Here's how the part is built. I have some questions about the finished solid (model axes, mm). A direction names the side the tool comes from. Give positions to 0.01 mm unless a question says otherwise; leave off trailing zeros. Order: outer loops, then holes, each group sorted by start corner. A loop starts at its lowest first (then second) coordinate and runs counter-clockwise, first axis right, second up.
from build123d import *

# Parameters (mm, degrees)
ESQUISSE1_W             = 22.3
ESQUISSE1_H             = 43
ESQUISSE1_R             = 2.45
BOSS_EXTRU_1_DEPTH      = 5
BOSS_EXTRU_2_START      = -2.47
ESQUISSE2_R             = 2.45
ESQUISSE2_R_2           = 0.7
BOSS_EXTRU_2_DEPTH      = 2.47
ESQUISSE3_W             = 4
ESQUISSE3_H             = 5
ESQUISSE3_W_2           = 3.94
BOSS_EXTRU_3_DEPTH      = 12.3
ESQUISSE4_R             = 0.7
ENL_V_MAT_EXTRU_1_DEPTH = 52.435201954
BOSS_EXTRU_4_DEPTH      = 2
BOSS_EXTRU_5_DEPTH      = 2
ESQUISSE7_R             = 0.7
BOSS_EXTRU_6_DEPTH      = 4
ESQUISSE8_R             = 0.7
ENL_V_MAT_EXTRU_3_DEPTH = 54.118546667


with BuildPart() as part:
    # Esquisse1 → Boss.-Extru.1 (new body)
    with BuildSketch(Plane.XY):
        with Locations((-11.15, -21.5)):
            Rectangle(ESQUISSE1_W, ESQUISSE1_H)
        with Locations((-6.15, -6.15)):
            Circle(ESQUISSE1_R, mode=Mode.SUBTRACT)
    extrude(amount=BOSS_EXTRU_1_DEPTH)

    # Esquisse2 → Boss.-Extru.2 (add)
    with BuildSketch(Plane.XY.offset(5).offset(BOSS_EXTRU_2_START)):
        with Locations((-6.15, -6.15)):
            Circle(ESQUISSE2_R)
        with Locations((-6.15, -6.15)):
            Circle(ESQUISSE2_R_2, mode=Mode.SUBTRACT)
    extrude(amount=BOSS_EXTRU_2_DEPTH)

    # Esquisse3 → Boss.-Extru.3 (add)
    with BuildSketch(Plane.XY.offset(5)):
        with Locations((-20.3, -40.5)):
            Rectangle(ESQUISSE3_W, ESQUISSE3_H)
        with Locations((-13.54, -40.5)):
            Rectangle(ESQUISSE3_W, ESQUISSE3_H)
        with Locations((-20.3, -12.82)):
            Rectangle(ESQUISSE3_W, ESQUISSE3_H)
        with Locations((-13.57, -12.82)):
            Rectangle(ESQUISSE3_W_2, ESQUISSE3_H)
    extrude(amount=BOSS_EXTRU_3_DEPTH)

    # Esquisse4 → Enlèv. mat.-Extru.1 (cut, through all)
    with BuildSketch(Plane.ZY.offset(22.3)):
        with Locations((11.15, -12.82)):
            Circle(ESQUISSE4_R)
        with Locations((11.15, -40.42)):
            Circle(ESQUISSE4_R)
    extrude(amount=-ENL_V_MAT_EXTRU_1_DEPTH, mode=Mode.SUBTRACT)

    # Esquisse5 → Boss.-Extru.4 (add)
    with BuildSketch(Plane.XZ.offset(43)):
        Polygon((-22.3, 17.3), (-11.54, 17.3), (0, 5), (0, 0), (-22.3, 0), align=None)
    extrude(amount=BOSS_EXTRU_4_DEPTH)

    # Esquisse6 → Boss.-Extru.5 (add)
    with BuildSketch(Plane(origin=(0, -10.32, 0), x_dir=(1, 0, 0), z_dir=(0, 1, 0))):
        Polygon((-22.3, -5), (-22.3, -17.3), (-11.6, -17.3), (0, -5), align=None)
    extrude(amount=BOSS_EXTRU_5_DEPTH)

    # Esquisse7 → Boss.-Extru.6 (add)
    with BuildSketch(Plane(origin=(0, 0, 0), x_dir=(0, 0, -1), z_dir=(1, 0, 0))):
        with BuildLine():
            Line((-11.15, -15.32), (0, -15.32))
            Line((0, -15.32), (0, -27.62))
            Line((0, -27.62), (-11.15, -27.62))
            ThreePointArc((-11.15, -27.62), (-17.3, -21.47), (-11.15, -15.32))
        make_face()
        with Locations(Location((-11.15, -21.47, 0), (0, 0, 90))):
            Circle(ESQUISSE7_R, mode=Mode.SUBTRACT)
    extrude(amount=BOSS_EXTRU_6_DEPTH)

    # Esquisse8 → Enlèv. mat.-Extru.3 (cut, through all)
    with BuildSketch(Plane(origin=(0, 0, 0), x_dir=(-1, 0, 0), z_dir=(0, 0, -1))):
        with Locations((17.3, -40)):
            Circle(ESQUISSE8_R)
        with Locations((5, -40)):
            Circle(ESQUISSE8_R)
        with Locations((5, -20)):
            Circle(ESQUISSE8_R)
        with Locations((17.3, -20)):
            Circle(ESQUISSE8_R)
    extrude(amount=-ENL_V_MAT_EXTRU_3_DEPTH, mode=Mode.SUBTRACT)


solid = part.part
Q1. If we section it at D-D on y = -12.82: List the corners of the cut face in (x, z) for me.
Filled sheet:
outline: (-22.3, 0) - (0, 0) - (0, 5) - (-11.6, 5) - (-11.6, 10.45) - (-15.54, 10.45) - (-15.54, 5) - (-18.3, 5) - (-18.3, 10.45) - (-22.3, 10.45) - close; (-22.3, 11.85) - (-18.3, 11.85) - (-18.3, 17.3) - (-22.3, 17.3) - close; (-15.54, 11.85) - (-11.6, 11.85) - (-11.6, 17.3) - (-15.54, 17.3) - close
Q2. If we section it at A-A on z = 1.5: List the corners of the cut face in (x, y) for me.
Filled sheet:
outline: (-22.3, -45) - (0, -45) - (0, -27.62) - (4, -27.62) - (4, -15.32) - (0, -15.32) - (0, 0) - (-22.3, 0) - close; hole circle Ø1.4 at (-17.3, -40); hole circle Ø1.4 at (-17.3, -20); hole circle Ø4.9 at (-6.15, -6.15); hole circle Ø1.4 at (-5, -40); hole circle Ø1.4 at (-5, -20)
Q3. If we section it at B-B on y = -21.47: List the corners of the cut face in (x, z) for me.
Filled sheet:
outline: (-22.3, 0) - (4, 0) - (4, 10.45) - (0, 10.45) - (0, 5) - (-22.3, 5) - close; (0, 11.85) - (4, 11.85) - (4, 17.3) - (0, 17.3) - close
Q4. Thinking about a two-plate mould opening in Y: for faces 5 (the face through (-11, 0, 2)), 6 (the face through (-9, -22, 0)), 7 (the face through (-4.909, -19.306, 2.465)), which applies, released by +Y, released by -Y, zero draft, split by the parting line, or undercut?
Filled sheet:
face 5: released by +Y
face 6: zero draft
face 7: undercut
Q5. For faces 1 (the face through (-11.6, -11.7, 11.1)), 2 (the face through (-11, -4, 5)), 3 (the face through (-17, -43, 11)), 4 (the face through (-20, -15.32, 11)), which set-ups out of +Z, -Z, +X, -X, +Y, -Y let a thin tool reach every point of the face, with its end or its side?
Filled sheet:
face 1: +Z, +X
face 2: +Z, +X, -X, +Y
face 3: +Z
face 4: +Z, -X
Q6. If we section it at C-C on x = -17.3: List the corners of the cut face in (y, z) for me.
Filled sheet:
outline: (-45, 0) - (-40.7, 0) - (-40.7, 5) - (-43, 5) - (-43, 17.3) - (-45, 17.3) - close; (-39.3, 0) - (-20.7, 0) - (-20.7, 5) - (-39.3, 5) - close; (-19.3, 0) - (0, 0) - (0, 5) - (-8.32, 5) - (-8.32, 17.3) - (-10.32, 17.3) - (-10.32, 5) - (-19.3, 5) - close
Q7. I need wall thicknesses on L1, parallel to Y at x = -17.3, z = 3.25; L2, parallel to Y at x = -21.25, z = 11.15; L3, parallel to X at y = -40, z = 2. Which ranges of each line are inside material? Lowest first, please.
Filled sheet:
L1: y = -45 to -40.7, -39.3 to -20.7, -19.3 to 0
L2: y = -45 to -41.12, -39.72 to -38, -15.32 to -13.52, -12.12 to -8.32
L3: x = -22.3 to -18, -16.6 to -5.7, -4.3 to 0
Q8. I'm going to push flat-ended pins straight in: P1, Ø3, axis at y = -39.5, z = 9.5, coming from the +X side; P2, Ø1.6, axis at y = -12.82, z = 11.15, coming from the +X side; P3, Ø6, axis at x = -7.5, z = 9, coming from the +Y side; P4, Ø1.3, axis at y = -21.47, z = 11.15, coming from the -X side. Where does each tip first touch, or does it pass through?
Filled sheet:
P1: stops at x = -11.54
P2: stops at x = -11.6
P3: stops at y = -8.32
P4: passes through
